Source: CAD feature listing. Evaluate the final solid. Frame: model axes, mm. Coordinates: 2 decimals unless noted, no trailing zeros. Loops run counter-clockwise (first coordinate to the right, second up) from the corner with the lowest first, then second, coordinate; pieces in that order, holes last. Notation, with made-up numbers: (80, 75.5) - (126, 75.5) arc R14 cw to (126, 83.5) - close; hole circle Ø9 at (6.25, 21). An arc over 180 degrees is marked (long way). Use one line per item in the form item = value. Start each with the question number.
from build123d import *

# Parameters (mm, degrees)
RESSALTO_EXTRUS_O1_DEPTH = 3


with BuildPart() as part:
    # Esboço1 → Ressalto-extrusão1 (new, symmetric)
    with BuildSketch(Plane.XY):
        with BuildLine():
            ThreePointArc((203, -7.4), (210.4, 0), (203, 7.4))
            Line((203, 7.4), (-203, 7.4))
            ThreePointArc((-203, 7.4), (-210.4, 0), (-203, -7.4))
            Line((-203, -7.4), (203, -7.4))
        make_face()
        with BuildLine():
            Line((-203, 5.4), (203, 5.4))
            ThreePointArc((203, 5.4), (208.4, 0), (203, -5.4))
            Line((203, -5.4), (-203, -5.4))
            ThreePointArc((-203, -5.4), (-208.4, 0), (-203, 5.4))
        make_face(mode=Mode.SUBTRACT)
    extrude(amount=RESSALTO_EXTRUS_O1_DEPTH, both=True)


solid = part.part
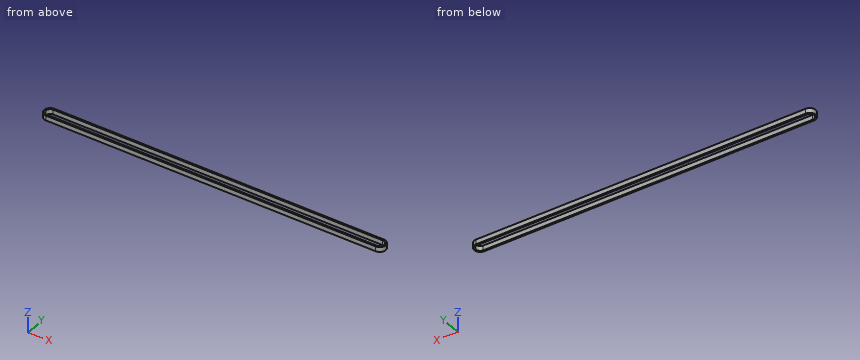
(1) Cut plane A-A, the plane y = 0. Output: boundary loops of the cut face in (x, z).
(2) Cut plane B-B, the plane z = 0.45. Output: boundary loops of the cut face in (x, y), plus the area to 3 significant figures.
(3) Cut plane C-C, the plane x = -35. Output: boundary loops of the cut face in (y, z), plus the area to 3 significant figures.
(4) Material intervals for line 1 (Y direction, x = 30.5, z = 2.1); line 2 (X direction, y = 0.5, z = -2.7); line 3 (X direction, y = -0.75, z = 1.8), sorted ascending.
(5) Contact query for flat-ended pins moving along their axis: pin 1 (1.5 mm diameter, centred on y = 4.5, z = 1.5, fed in from -X); pin 2 (1 mm diameter, centred on y = 2.5, z = -1.5, fed in from +X). Output: stop coordinate, or through.
Recorded:
q1.outline = (-210.4, -3) - (-208.4, -3) - (-208.4, 3) - (-210.4, 3) - close; (208.4, -3) - (210.4, -3) - (210.4, 3) - (208.4, 3) - close
q2.outline = (-203, -7.4) - (203, -7.4) arc R7.4 ccw to (203, 7.4) - (-203, 7.4) arc R7.4 ccw to start; hole (-203, -5.4) - (203, -5.4) arc R5.4 ccw to (203, 5.4) - (-203, 5.4) arc R5.4 ccw to start
q2.area = 1,700 mm²
q3.outline = (-7.4, -3) - (-5.4, -3) - (-5.4, 3) - (-7.4, 3) - close; (5.4, -3) - (7.4, -3) - (7.4, 3) - (5.4, 3) - close
q3.area = 24.0 mm²
q4.line_1 = -7.4 to -5.4, 5.4 to 7.4
q4.line_2 = -210.38 to -208.38, 208.38 to 210.38
q4.line_3 = -210.36 to -208.35, 208.35 to 210.36
q5.pin_1 = -209.38
q5.pin_2 = 210.12
